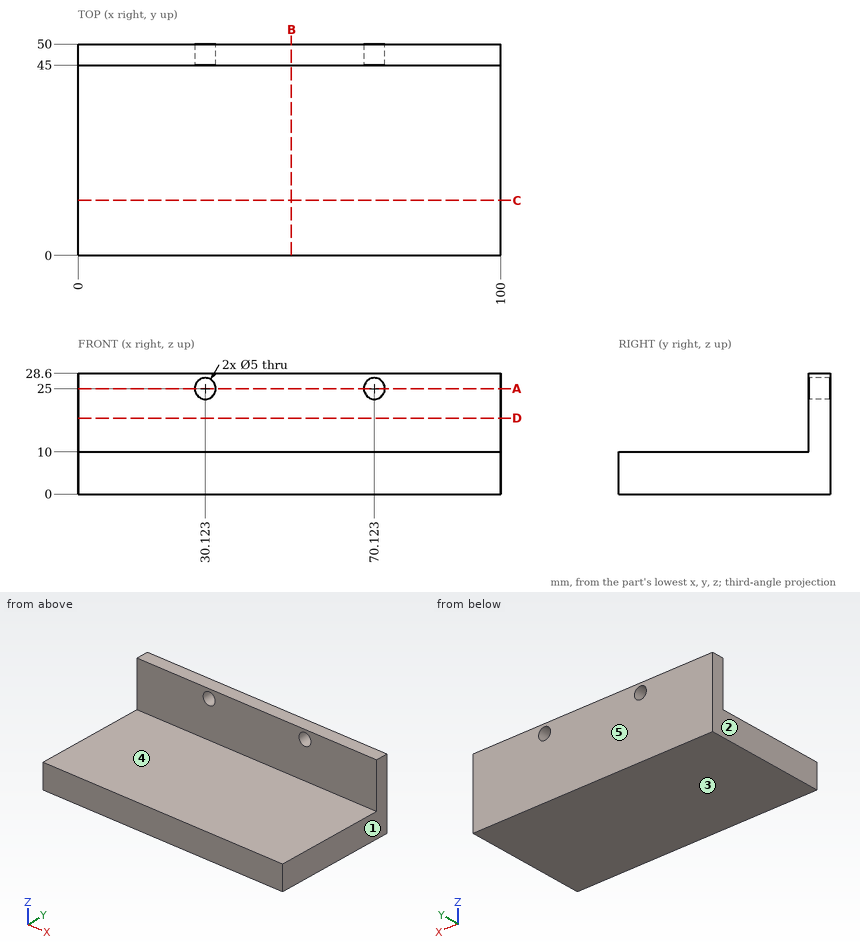
Verification items for this drawing (mm, ordinates from the low corner). A direction names the side the tool comes from. Give positions to 0.01 mm unless a question says otherwise; leave off trailing zeros. Write each loop counter-clockwise with the first axis right and the second up, starting at its lowest first coordinate (ties: lowest second). Pieces come first, ordered by that corner, then holes. Notation, with made-up numbers: (-7, 43.5) - (26, 43.5) arc R19 ccw to (26, 76.5) - close; hole circle Ø8 at (83, 5). An arc over 180 degrees is marked (long way). Answer as a JSON object with one key per item and string values. Group by question number.
1) Access from +Z, -Z, +X, -X, +Y, -Y to the whole of each face (thin tool, end or side, straight path). Record for the marked faces 4 and 5.
2) Release check for a two-part mould opening along X. For the marked faces 1, 2 and 3 record: pulls with the +X half, pulls with the -X half, needs draft (parallel to the pull), parting line crosses it, or undercut.
3) Sectioned sample at B-B (x = 50.5). Record the cut outline in (y, z).
4) Depth check by flat-ended pin: P1, Ø6, axis at x = 50.5, y = 34.5, coming from the -Z side; P2, Ø8, axis at x = 28.5, z = 14.5, coming from the -Y side; P3, Ø6, axis at x = 77, y = 11.5, coming from the +Z side. Enter the tip coordinate at first touch or a pass-through.
5) Thickness scan on probe 1 along Z at (x, y) = (38.5, 36.5); probe 2 along Y at (x, z) = (45, 16.5). Record the ranges inside material, lowest first. Write a range as from..to.
6) Sectioned sample at C-C (y = 13). Record the cut outline in (x, z), then the cut area to 3 significant figures.
7) Sectioned sample at A-A (z = 25). Record the cut outline in (x, y), then the cut area to 3 significant figures.
8) Sectioned sample at D-D (z = 18). Record the cut outline in (x, y).
Geometry results:
{
 "1": {"face 4": "+Z, +X, -X, -Y", "face 5": "+Z, -Z, +X, -X, +Y"},
 "2": {"face 1": "pulls with the +X half", "face 2": "pulls with the -X half", "face 3": "needs draft"},
 "3": {"outline": "(0, 0) - (50, 0) - (50, 28.6) - (45, 28.6) - (45, 10) - (0, 10) - close"},
 "4": {"P1": "stops at z = 0", "P2": "stops at y = 45", "P3": "stops at z = 10"},
 "5": {"probe 1": "z = 0..10", "probe 2": "y = 45..50"},
 "6": {"outline": "(0, 0) - (100, 0) - (100, 10) - (0, 10) - close", "area": "1,000 mm^2"},
 "7": {"outline": "(0, 45) - (27.62, 45) - (27.62, 50) - (0, 50) - close; (32.62, 45) - (67.62, 45) - (67.62, 50) - (32.62, 50) - close; (72.62, 45) - (100, 45) - (100, 50) - (72.62, 50) - close", "area": "450 mm^2"},
 "8": {"outline": "(0, 45) - (100, 45) - (100, 50) - (0, 50) - close"}
}
